Check sheet for the modelled part. Datum: model origin and axes. Units: mm. A direction names the side the tool comes from. Coordinates: 2 decimals unless noted, no trailing zeros. Loops run counter-clockwise (first coordinate to the right, second up) from the corner with the lowest first, then second, coordinate; pieces in that order, holes last. Notation, with made-up numbers: M -1,60 L 24,60 A23 cw 24,81 Z; hole C 12.5,25.25 d1. An arc over 180 degrees is marked long. Answer as CSV lines item,"result". Start each with the question number.
from build123d import *

# Parameters (mm, degrees)
EXTRUDE_THIN1_DEPTH             = 76.2
TAP_DRILL_FOR_M5X0_8_TAP1_D     = 4.2
TAP_DRILL_FOR_M5X0_8_TAP1_DEPTH = 11.938
TAP_DRILL_FOR_M5X0_8_TAP1_TIP   = 1.2618073
SKETCH4_R                       = 19.0627
CUT_EXTRUDE1_DEPTH              = 198.182581951


with BuildPart() as part:
    # Sketch1 → Extrude-Thin1 (new body)
    with BuildSketch(Plane.XY):
        Polygon((0, 0), (127, 0), (127, 127), (130.175, 127), (130.175, -3.175), (0, -3.175), align=None)
    extrude(amount=EXTRUDE_THIN1_DEPTH)

    # Tap Drill for M5x0.8 Tap1
    with Locations(Plane(origin=(130.175, 0, 0), x_dir=(0, 0, -1), z_dir=(1, 0, 0))):
        with Locations((-14.5, 85.5125), (-61.7, 38.3125), (-61.7, 85.5125), (-14.5, 38.3125)):
            Hole(TAP_DRILL_FOR_M5X0_8_TAP1_D / 2, depth=TAP_DRILL_FOR_M5X0_8_TAP1_DEPTH)
            with Locations((0, 0, -(TAP_DRILL_FOR_M5X0_8_TAP1_DEPTH + TAP_DRILL_FOR_M5X0_8_TAP1_TIP / 2))):  # 118° drill point
                Cone(0, TAP_DRILL_FOR_M5X0_8_TAP1_D / 2, TAP_DRILL_FOR_M5X0_8_TAP1_TIP, mode=Mode.SUBTRACT)

    # Sketch4 → Cut-Extrude1 (cut, through all)
    with BuildSketch(Plane(origin=(130.175, 0, 0), x_dir=(0, 0, -1), z_dir=(1, 0, 0))):
        with Locations((-38.1, 61.9125)):
            Circle(SKETCH4_R)
    extrude(amount=-CUT_EXTRUDE1_DEPTH, mode=Mode.SUBTRACT)


solid = part.part
Item 1: Material ranges on line 1 (Y direction, x = 129.5, z = 61.7) (1 decimal); line 2 (Y direction, x = 128, z = 61) (3 decimals); line 3 (Y direction, x = 128.1, z = 38.1) (3 decimals), recorded low to high. Write a range as from..to.
Item 2: Release check for a two-part mould opening along Y. For faces 3 (the face through (66, -3.175, 38)), 4 (the face through (127, 48, 54)), 5 (the face through (128.565, 83.462, 14.045)) record: released by +Y, released by -Y, zero draft, split by the parting line, or undercut.
Item 3: Set-up check for faces 1 (the face through (63, 0, 38)), 2 (the face through (130.175, 77, 54)): record each of +Z, -Z, +X, -X, +Y, -Y from which the full face is reachable in a straight line by a thin tool's end or side.
Item 4: Sectioned sample at D-D, the plane z = 6. Record the boundary of the cut face in (x, y) (3 decimals), and give its area (3 significant figures).
Item 5: Go/stop test with a flat-tipped pin: pin 1 (10 mm diameter, centred on y = 95, z = 53.5, fed in from -X). Record where the tip stops, or that it passes through.
Item 6: Sectioned sample at C-C, the plane y = 55. Record the boundary of the cut face in (x, z) (3 decimals).
Item 7: Sectioned sample at B-B, the plane z = 14.5. Record the boundary of the cut face in (x, y) (1 decimal), and give its area (3 significant figures).
Item 8: Sectioned sample at A-A, the plane z = 38.1. Record the boundary of the cut face in (x, y) (3 decimals).
Reply:
1,line 1,"-3.2..36.2, 40.4..83.4, 87.6..127"
1,line 2,"-3.175..36.333, 40.292..83.533, 87.492..127"
1,line 3,"-3.175..42.85, 80.975..127"
2,face 3,"released by -Y"
2,face 4,"zero draft"
2,face 5,"undercut"
3,face 1,"+Z, -Z, -X, +Y"
3,face 2,"+Z, -Z, +X, +Y, -Y"
4,outline,"M 0,-3.175 L 130.175,-3.175 L 130.175,127 L 127,127 L 127,0 L 0,0 Z"
4,area,"817 mm²"
5,pin 1,"x = 127"
6,outline,"M 127,0 L 130.175,0 L 130.175,20.335 L 127,20.335 Z; M 127,55.865 L 130.175,55.865 L 130.175,76.2 L 127,76.2 Z"
7,outline,"M 0,-3.2 L 130.2,-3.2 L 130.2,36.2 L 127,36.2 L 127,0 L 0,0 Z; M 127,40.4 L 130.2,40.4 L 130.2,83.4 L 127,83.4 Z; M 127,87.6 L 130.2,87.6 L 130.2,127 L 127,127 Z"
7,area,"790 mm²"
8,outline,"M 0,-3.175 L 130.175,-3.175 L 130.175,42.85 L 127,42.85 L 127,0 L 0,0 Z; M 127,80.975 L 130.175,80.975 L 130.175,127 L 127,127 Z"
